Work out the finished part from the listing and answer in its coordinate system (mm). A direction names the side the tool comes from. Coordinates: 2 decimals unless noted, no trailing zeros. Write each loop counter-clockwise with the first axis right and the second up, starting at its lowest first coordinate (ties: lowest second). Pieces come first, ordered by that corner, then holes. Notation, with made-up numbers: (-32.75, -11.75) - (3.25, -11.75) arc R20 cw to (3.25, 24.25) - close; hole circle Ø1 at (71, 44.5). An arc over 180 degrees is marked (long way). Use one line per item in the form item = value. Start each with the question number.
Item 1: A cutting plane is placed at A-A (x = 0). Write down the section's boundary in (y, z), then the cut area to 3 significant figures.
Item 2: A cutting plane is placed at B-B (y = -11). Write down the section's boundary in (x, z), then the cut area to 3 significant figures.
Item 3: Determine the mould class of faces 5 (the cylindrical face through (-1.322, -1.972, 1.145)), 6 (the flat face through (-49, -11, -85)), 7 (the flat face through (1, 0, -47)) for opening direction X: released by +X, released by -X, zero draft, split by the parting line, or undercut.
Item 4: For faces 1 (the flat face through (-36, -11, -74)), 2 (the flat face through (-17, -2.5, -1)), 3 (the flat face through (0, -4, 0)), 4 (the flat face through (36, -12, -74)), determine the directions among +Z, -Z, +X, -X, +Y, -Y from which every point of the face is accessible in a straight line to the end or side of a thin tool.
Item 5: A cutting plane is placed at D-D (z = -83). Write down the section's boundary in (x, y), then the cut area to 3 significant figures.
Item 6: Given pin 1 (3.5 mm diameter, centred on x = -15.5, z = 0, fed in from +Y); pin 2 (12 mm diameter, centred on x = 37, z = -70.5, fed in from -Y); pin 3 (1 mm diameter, centred on y = -6.5, z = -39, fed in from -X); pin 4 (1.6 mm diameter, centred on x = -16, z = 0, fed in from +Y), each flat-ended and moving along its own axis, determine where each tip first touches the part or whether it passes through.
Item 7: A cutting plane is placed at C-C (z = 7.1). Write down the section's boundary in (x, y).
Item 8: Consider probe 1 along Z at (x, y) = (0, -10.75); probe 2 along Z at (x, y) = (-7.75, -1.9); probe 3 along Y at (x, z) = (1.5, -44). Determine where each line is inside the solid, lowest interval first.
from build123d import *

# Parameters (mm, degrees)
F0_R          = 19
F0_R_2        = 1.5
F0_R_3        = 6.1
F1_DEPTH      = 4
F2_R          = 24
F2_R_2        = 19
F3_DEPTH      = 27
F5_DEPTH      = 25
F6_R          = 2.65
F7_DEPTH      = 2.5
F8_W          = 24
F8_H          = 54
F9_DEPTH      = 25
F10_W         = 25
F10_H         = 20
F11_DEPTH     = 25
F13_W         = 25
F13_H         = 20
F14_DEPTH     = 25
F15_R         = 2
F17_DEPTH     = 25
F18_DEPTH     = 25
F19_T1_DEPTH  = 25
F19_T3_DEPTH  = 21
F19_T5_DEPTH  = 23
F19_T7_DEPTH  = 21
F19_T12_DEPTH = 87
F19_S13_R     = 24
F19_T14_DEPTH = 45
F19_T18_DEPTH = 87
F19_S19_R     = 24
F19_T20_DEPTH = 45
F19_T22_ANGLE = 90
F19_T24_ANGLE = 90
F19_T26_ANGLE = 90
F19_T28_ANGLE = 90


# Not quite as in the source:
# - a fillet or chamfer that OpenCascade refuses, or shapes differently, is made with other operations: its cross-section is extruded or revolved along the edge and cut away or added


with BuildPart() as f1:
    # F0 (on Front) → F1 (new body)
    with BuildSketch(Plane.XZ):
        Circle(F0_R)
        with Locations((-7.75, -13.4233937587)):
            Circle(F0_R_2, mode=Mode.SUBTRACT)
        with Locations((7.75, -13.4233937587)):
            Circle(F0_R_2, mode=Mode.SUBTRACT)
        with Locations((-15.5, 0)):
            Circle(F0_R_2, mode=Mode.SUBTRACT)
        with Locations((-7.75, 13.4233937587)):
            Circle(F0_R_2, mode=Mode.SUBTRACT)
        with Locations((0, 7.1)):
            Circle(F0_R_3, mode=Mode.SUBTRACT)
        with BuildLine():
            ThreePointArc((14, 0), (15.5, 1.5), (17, 0))
            ThreePointArc((17, 0), (15.5, -1.5), (14, 0))
        make_face(mode=Mode.SUBTRACT)
        with Locations((7.75, 13.4233937587)):
            Circle(F0_R_2, mode=Mode.SUBTRACT)
    extrude(amount=F1_DEPTH)

    # F2 (on Front) → F3 (join)
    with BuildSketch(Plane.XZ):
        Circle(F2_R)
        Circle(F2_R_2, mode=Mode.SUBTRACT)
    extrude(amount=F3_DEPTH)

    # F4 (on face) → F5 (join)
    with BuildSketch(Plane(origin=(0, 0, 0), x_dir=(-1, 0, 0), z_dir=(0, 1, 0))):
        with BuildLine():
            Line((24, -40), (24, 0))
            ThreePointArc((24, 0), (0, -24), (-24, 0))
            Line((-24, 0), (-24, -40))
            Line((-24, -40), (0, -40))
            Line((0, -40), (24, -40))
        make_face()
    extrude(amount=-F5_DEPTH)

    # F6 (on face) → F7 (cut)
    with BuildSketch(Plane(origin=(0, 0, 0), x_dir=(-1, 0, 0), z_dir=(0, 1, 0))):
        with Locations((-7.75, 13.4233937587)):
            Circle(F6_R)
        with Locations((7.75, 13.4233937587)):
            Circle(F6_R)
        with Locations((-15.5, 0)):
            Circle(F6_R)
        with Locations((15.5, 0)):
            Circle(F6_R)
    extrude(amount=-F7_DEPTH, mode=Mode.SUBTRACT)

    # F8 (on face) → F9 (join, through all)
    with BuildSketch(Plane.XZ.offset(25)):
        with Locations((12, -67)):
            Rectangle(F8_W, F8_H)
        with Locations((-12, -67)):
            Rectangle(F8_W, F8_H)
    extrude(amount=-F9_DEPTH)

    # F10 (on face) → F11 (join)
    with BuildSketch(Plane.YZ.offset(24)):
        with Locations((-12.5, -84)):
            Rectangle(F10_W, F10_H)
    extrude(amount=F11_DEPTH)

    # F13 (on face) → F14 (join)
    with BuildSketch(Plane(origin=(-24, 0, 0), x_dir=(0, -1, 0), z_dir=(-1, 0, 0))):
        with Locations((12.5, -84)):
            Rectangle(F13_W, F13_H)
    extrude(amount=F14_DEPTH)

    # F15
    f15_edges = [f1.edges().sort_by_distance(p)[0] for p in [
        (49, -12.5, -74),
        (-49, -12.5, -74),
    ]]
    fillet(f15_edges, radius=F15_R)

    # F16 (on face) → F17 (cut)
    with BuildSketch(Plane(origin=(0, 0, -94), x_dir=(1, 0, 0), z_dir=(0, 0, -1))):
        with BuildLine():
            ThreePointArc((-38.75, 12.5), (-41.5, 15.25), (-44.25, 12.5))
            Line((-44.25, 12.5), (-38.75, 12.5))
        make_face()
        with BuildLine():
            Line((-38.75, 12.5), (-44.25, 12.5))
            ThreePointArc((-44.25, 12.5), (-41.5, 9.75), (-38.75, 12.5))
        make_face()
    extrude(amount=-F17_DEPTH, mode=Mode.SUBTRACT)

    # F12 (on face) → F18 (cut)
    with BuildSketch(Plane.XY.offset(-74)):
        with BuildLine():
            ThreePointArc((38.75, -12.5), (41.5, -15.25), (44.25, -12.5))
            Line((44.25, -12.5), (38.75, -12.5))
        make_face()
        with BuildLine():
            Line((38.75, -12.5), (44.25, -12.5))
            ThreePointArc((44.25, -12.5), (41.5, -9.75), (38.75, -12.5))
        make_face()
    extrude(amount=-F18_DEPTH, mode=Mode.SUBTRACT)

    # F19: fillet of radius 2 on 10 edges, made by hand

    # F19_s2 → F19_t1 (join)
    with BuildSketch(Plane.XZ):
        with BuildLine():
            ThreePointArc((24, -72), (24.5857864376, -73.4142135624), (26, -74))
            Line((26, -74), (24, -74))
            Line((24, -74), (24, -72))
        make_face()
        with BuildLine():
            ThreePointArc((-26, -74), (-24.5857864376, -73.4142135624), (-24, -72))
            Line((-24, -72), (-24, -74))
            Line((-24, -74), (-26, -74))
        make_face()
    extrude(amount=F19_T1_DEPTH)

    # F19_s4 → F19_t3 (cut)
    with BuildSketch(Plane.YZ.offset(-47)):
        with BuildLine():
            ThreePointArc((-23, -74), (-24.4142135624, -74.5857864376), (-25, -76))
            Line((-25, -76), (-25, -74))
            Line((-25, -74), (-23, -74))
        make_face()
    extrude(amount=F19_T3_DEPTH, mode=Mode.SUBTRACT)

    # F19_s6 → F19_t5 (cut)
    with BuildSketch(Plane.XY.offset(-99)):
        with BuildLine():
            ThreePointArc((-49, -23), (-48.4142135624, -24.4142135624), (-47, -25))
            Line((-47, -25), (-49, -25))
            Line((-49, -25), (-49, -23))
        make_face()
        with BuildLine():
            ThreePointArc((49, -23), (48.4142135624, -24.4142135624), (47, -25))
            Line((47, -25), (49, -25))
            Line((49, -25), (49, -23))
        make_face()
    extrude(amount=F19_T5_DEPTH, mode=Mode.SUBTRACT)

    # F19_s8 → F19_t7 (cut)
    with BuildSketch(Plane.YZ.offset(26)):
        with BuildLine():
            ThreePointArc((-23, -74), (-24.4142135624, -74.5857864376), (-25, -76))
            Line((-25, -76), (-25, -74))
            Line((-25, -74), (-23, -74))
        make_face()
    extrude(amount=F19_T7_DEPTH, mode=Mode.SUBTRACT)


with BuildPart() as f19_tool10:
    # F19_s11 → F19_t12 (new body)
    with BuildSketch(Plane.XY.offset(15)):
        with BuildLine():
            ThreePointArc((24, -23), (23.4142135624, -24.4142135624), (22, -25))
            Line((22, -25), (24, -25))
            Line((24, -25), (24, -23))
        make_face()
    extrude(amount=-F19_T12_DEPTH)

    # F19_s13 → F19_t14 (cut, symmetric)
    with BuildSketch(Plane.XZ.offset(24)):
        Circle(F19_S13_R)
    extrude(amount=F19_T14_DEPTH, both=True, mode=Mode.SUBTRACT)


with BuildPart() as f1_1:
    add(f1.part)

    # F19_t9: cut F19_tool10
    add(f19_tool10.part, mode=Mode.SUBTRACT)


with BuildPart() as f19_tool16:
    # F19_s17 → F19_t18 (new body)
    with BuildSketch(Plane.XY.offset(-72)):
        with BuildLine():
            ThreePointArc((-24, -23), (-23.4142135624, -24.4142135624), (-22, -25))
            Line((-22, -25), (-24, -25))
            Line((-24, -25), (-24, -23))
        make_face()
    extrude(amount=F19_T18_DEPTH)

    # F19_s19 → F19_t20 (cut, symmetric)
    with BuildSketch(Plane.XZ.offset(24)):
        Circle(F19_S19_R)
    extrude(amount=F19_T20_DEPTH, both=True, mode=Mode.SUBTRACT)


with BuildPart() as f1_2:
    add(f1_1.part)

    # F19_t15: cut F19_tool16
    add(f19_tool16.part, mode=Mode.SUBTRACT)

    # F19_s21 → F19_t22 (revolve, cut)
    with BuildSketch(Plane.XY.offset(-76)):
        with BuildLine():
            ThreePointArc((-49, -23), (-48.4142135624, -24.4142135624), (-47, -25))
            Line((-47, -25), (-49, -25))
            Line((-49, -25), (-49, -23))
        make_face()
    revolve(axis=Axis((-47, -25, -76), (0, 1, 0)), revolution_arc=F19_T22_ANGLE, mode=Mode.SUBTRACT)

    # F19_s23 → F19_t24 (revolve, cut)
    with BuildSketch(Plane.YZ.offset(47)):
        with BuildLine():
            ThreePointArc((-23, -74), (-24.4142135624, -74.5857864376), (-25, -76))
            Line((-25, -76), (-25, -74))
            Line((-25, -74), (-23, -74))
        make_face()
    revolve(axis=Axis((47, -25, -76), (0, 1, 0)), revolution_arc=F19_T24_ANGLE, mode=Mode.SUBTRACT)

    # F19_s25 → F19_t26 (revolve, cut)
    with BuildSketch(Plane.XY.offset(-72)):
        with BuildLine():
            ThreePointArc((22, -25), (23.4142135624, -24.4142135624), (24, -23))
            Line((24, -23), (24, -25))
            Line((24, -25), (22, -25))
        make_face()
    revolve(axis=Axis((26, -25, -72), (0, -1, 0)), revolution_arc=F19_T26_ANGLE, mode=Mode.SUBTRACT)

    # F19_s27 → F19_t28 (revolve, cut)
    with BuildSketch(Plane.YZ.offset(-26)):
        with BuildLine():
            ThreePointArc((-23, -74), (-24.4142135624, -74.5857864376), (-25, -76))
            Line((-25, -76), (-25, -74))
            Line((-25, -74), (-23, -74))
        make_face()
    revolve(axis=Axis((-26, -25, -72), (0, -1, 0)), revolution_arc=F19_T28_ANGLE, mode=Mode.SUBTRACT)


solid = f1_2.part
Answer:
q1.outline = (-27, -24) - (-25, -24) - (-25, -94) - (0, -94) - (0, 1) - (-4, 1) - (-4, -19) - (-27, -19) - close; (-27, 19) - (-4, 19) - (-4, 13.2) - (0, 13.2) - (0, 24) - (-27, 24) - close
q1.area = 2,120 mm²
q2.outline = (-49, -94) - (-43.8, -94) - (-43.8, -74) - (-47, -74) arc R2 ccw to (-49, -76) - close; (-39.2, -94) - (39.2, -94) - (39.2, -74) - (26, -74) arc R2 cw to (24, -72) - (24, 0) arc R24 ccw to (-24, 0) - (-24, -72) arc R2 cw to (-26, -74) - (-39.2, -74) - close; (43.8, -94) - (49, -94) - (49, -76) arc R2 ccw to (47, -74) - (43.8, -74) - close; hole circle Ø38 at (0, 0)
q2.area = 5,100 mm²
q3.face_5 = undercut
q3.face_6 = released by -X
q3.face_7 = zero draft
q4.face_1 = +Z, -X, +Y, -Y
q4.face_2 = +Y
q4.face_3 = -Y
q4.face_4 = +Z, +X, +Y, -Y
q5.outline = (-49, -23) arc R2 ccw to (-47, -25) - (47, -25) arc R2 ccw to (49, -23) - (49, 0) - (-49, 0) - close; hole circle Ø5.5 at (-41.5, -12.5); hole circle Ø5.5 at (41.5, -12.5)
q5.area = 2,400 mm²
q6.pin_1 = -2.5
q6.pin_2 = -25
q6.pin_3 = -24
q6.pin_4 = through
q7.outline = (-22.93, -27) - (-17.62, -27) - (-17.62, -4) - (-6.1, -4) - (-6.1, 0) - (-22.93, 0) - close; (6.1, -4) - (17.62, -4) - (17.62, -27) - (22.93, -27) - (22.93, 0) - (6.1, 0) - close
q8.probe_1 = -94 to -19, 19 to 24
q8.probe_2 = -94 to -14.92, -11.92 to 10.77, 16.07 to 22.71
q8.probe_3 = -25 to 0
